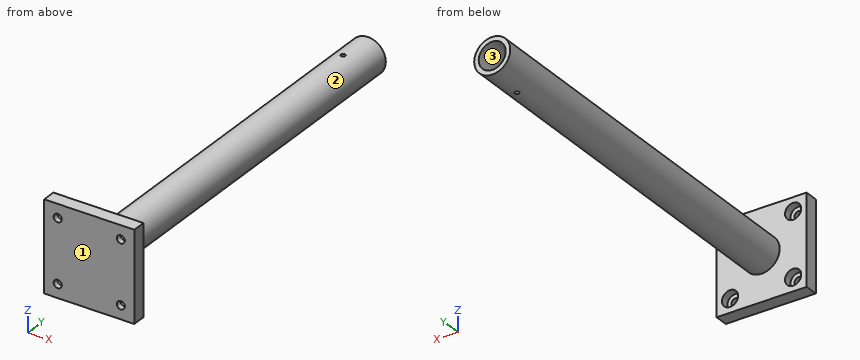
```python
from build123d import *

# Parameters (mm, degrees)
SKETCH4_W           = 100
SKETCH4_H           = 100
BOSS_EXTRUDE4_DEPTH = 15
SKETCH5_R           = 20
SKETCH5_R_2         = 15
BOSS_EXTRUDE5_DEPTH = 442
SKETCH8_R           = 2.5
CUT_EXTRUDE2_DEPTH  = 334
SKETCH9_R           = 4.5
CUT_EXTRUDE3_DEPTH  = 334
SKETCH10_R          = 9
CUT_EXTRUDE4_DEPTH  = 8.8


with BuildPart() as part:
    # Sketch4 → Boss-Extrude4 (new body)
    with BuildSketch(Plane(origin=(0, 0, 0), x_dir=(1, 0, 0), z_dir=(0, 1, 0))):
        with Locations((50, 50)):
            Rectangle(SKETCH4_W, SKETCH4_H)
    extrude(amount=BOSS_EXTRUDE4_DEPTH)

    # Sketch5 → Boss-Extrude5 (add)
    with BuildSketch(Plane(origin=(0, 15, 0), x_dir=(1, 0, 0), z_dir=(0, 1, 0))):
        with Locations((50, 50)):
            Circle(SKETCH5_R)
        with Locations((50, 50)):
            Circle(SKETCH5_R_2, mode=Mode.SUBTRACT)
    extrude(amount=BOSS_EXTRUDE5_DEPTH)

    # Sketch8 → Cut-Extrude2 (cut)
    with BuildSketch(Plane.XY):
        with Locations((50, 416.5)):
            Circle(SKETCH8_R)
    extrude(amount=-CUT_EXTRUDE2_DEPTH, mode=Mode.SUBTRACT)

    # Sketch9 → Cut-Extrude3 (cut)
    with BuildSketch(Plane(origin=(0, 15, 0), x_dir=(1, 0, 0), z_dir=(0, 1, 0))):
        with Locations((15, 85)):
            Circle(SKETCH9_R)
        with Locations((85, 85)):
            Circle(SKETCH9_R)
        with Locations((85, 15)):
            Circle(SKETCH9_R)
        with Locations((15, 15)):
            Circle(SKETCH9_R)
    extrude(amount=-CUT_EXTRUDE3_DEPTH, mode=Mode.SUBTRACT)

    # Sketch10 → Cut-Extrude4 (cut)
    with BuildSketch(Plane(origin=(0, 15, 0), x_dir=(1, 0, 0), z_dir=(0, 1, 0))):
        with Locations((15, 85)):
            Circle(SKETCH10_R)
        with Locations((85, 85)):
            Circle(SKETCH10_R)
        with Locations((85, 15)):
            Circle(SKETCH10_R)
        with Locations((15, 15)):
            Circle(SKETCH10_R)
    extrude(amount=-CUT_EXTRUDE4_DEPTH, mode=Mode.SUBTRACT)


solid = part.part
```
Source: CAD feature listing. Evaluate the final solid. Frame: model axes, mm. Face numbers are marked on the shaded views. Coordinates: 2 decimals unless noted, no trailing zeros. Loops run counter-clockwise (first coordinate to the right, second up) from the corner with the lowest first, then second, coordinate; pieces in that order, holes last. Notation, with made-up numbers: (50.5, 78) -> (107.5, 78) arc R16 cw to (107.5, 88) -> close; hole circle Ø1 at (16, 57). An arc over 180 degrees is marked (long way). One line per item, written item: value. Start each with the question number.
Q1. Contact query for flat-ended pins moving along their axis: P1, Ø14.5, axis at x = 19, z = -14, coming from the +Y side; P2, Ø16, axis at x = 85, z = -85, coming from the +Y side; P3, Ø5, axis at x = 31.5, y = 165, coming from the +Z side; P4, Ø16, axis at x = 15, z = -15, coming from the -Y side. Output: stop coordinate, or through.
Q2. Section query B-B, the plane y = 175.5. Return the cut outline in (x, z).
Q3. Mould query, pull axis Z, two halves, no side actions, for the marked faces 1, 2 and 3. Classes: pulls with the +Z half, pulls with the -Z half, needs draft (parallel to the pull), parting line crosses it, or undercut.
Q4. Section query A-A, the plane z = -15. Return the cut outline in (x, y), and give its area (3 significant figures).
Q5. Line query: line 1 along X through (y, z) = (11, -15); line 2 along Z through (x, y) = (85, 10); line 3 along X through (y, z) = (3, -85). Output: solid intervals per line, ascending.
Q6. Section query C-C, the plane z = -50. Return the cut outline in (x, y).
Results:
1. P1: y = 15
1. P2: y = 6.2
1. P3: z = -38
1. P4: y = 0
2. outline: circle Ø40 at (50, -50); hole circle Ø30 at (50, -50)
3. face 1: needs draft
3. face 2: parting line crosses it
3. face 3: undercut
4. outline: (0, 0) -> (10.5, 0) -> (10.5, 6.2) -> (6, 6.2) -> (6, 15) -> (0, 15) -> close; (19.5, 0) -> (80.5, 0) -> (80.5, 6.2) -> (76, 6.2) -> (76, 15) -> (24, 15) -> (24, 6.2) -> (19.5, 6.2) -> close; (89.5, 0) -> (100, 0) -> (100, 15) -> (94, 15) -> (94, 6.2) -> (89.5, 6.2) -> close
4. area: 1,070 mm^2
5. line 1: 0 to 6, 24 to 76, 94 to 100
5. line 2: -100 to -94, -76 to -24, -6 to 0
5. line 3: 0 to 10.5, 19.5 to 80.5, 89.5 to 100
6. outline: (0, 0) -> (100, 0) -> (100, 15) -> (70, 15) -> (70, 457) -> (65, 457) -> (65, 15) -> (35, 15) -> (35, 457) -> (30, 457) -> (30, 15) -> (0, 15) -> close
